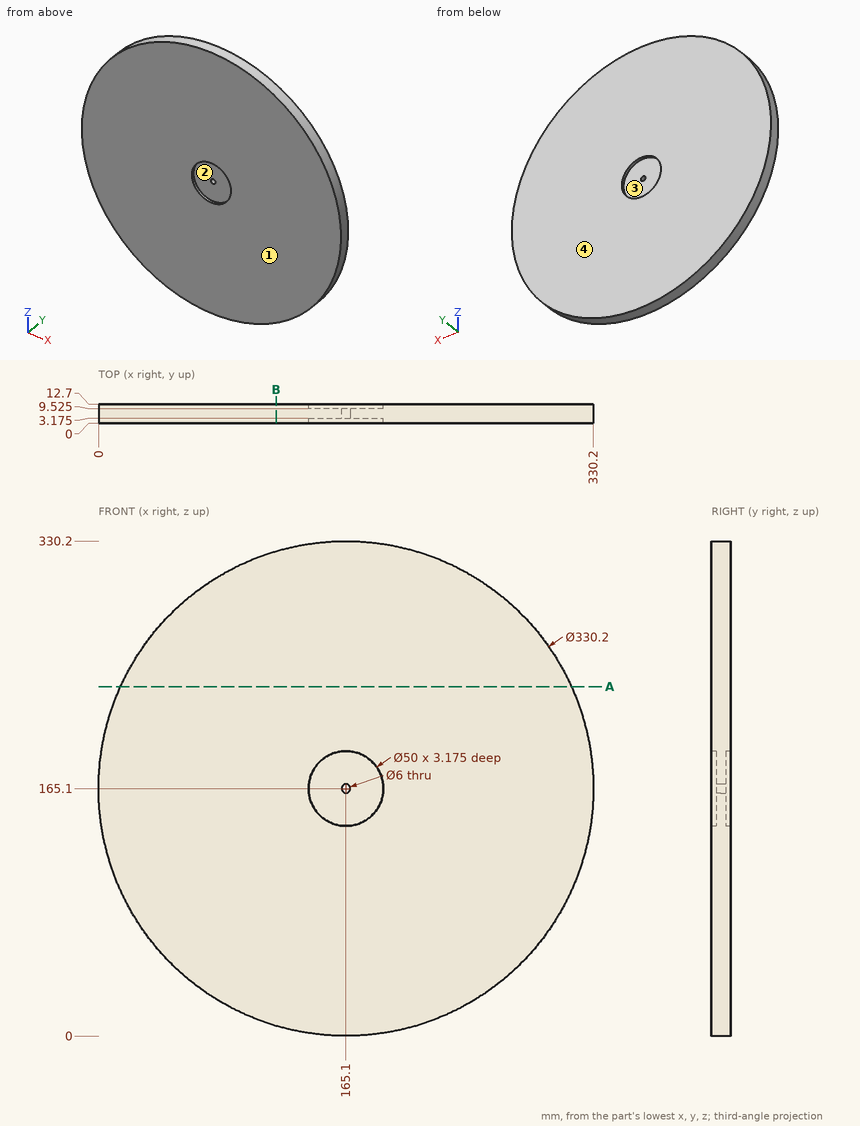
Part print with two shaded views. Sizes in mm from the minimum x, y, z corner. A direction names the side the tool comes from. Round coordinates to 2 decimals unless told otherwise and drop trailing zeros. Write each loop counter-clockwise with the first axis right and the second up, starting at its lowest first coordinate (ties: lowest second). Pieces come first, ordered by that corner, then holes. Notation, with made-up numbers: M -6,45 L 16,45 A25 cw 16,83 Z; hole C -13,-32 d7. An arc over 180 degrees is marked long. Put each result on its own line as item: value. Start each with the question number.
1) Pull direction X, two halves, no side cores. Call the marked faces 3 and 4: pulls with the +X half, pulls with the -X half, needs draft (parallel to the pull), parting line crosses it, or undercut.
2) Drill centre lines: probe 1 along X at (y, z) = (10.5, 165.1); probe 2 along X at (y, z) = (7.75, 165.1); probe 3 along Z at (x, y) = (216, 2). Where is each one in solid material? Low to high. Write a range as [from, to].
3) Pin check, flat tips, straight feed: pin 1 Ø6 at (y, z) = (2, 140.5) entering from +X; pin 2 Ø5 at (x, y) = (194.5, 4) entering from +Z; pin 3 Ø6 at (x, y) = (191.5, 3.5) entering from +Z; pin 4 Ø5.5 at (x, z) = (165.1, 165.1) entering from +Y. Stop position of each tip, or through.
4) Saw through at A-A, the plane z = 233. Write the cut outline in (x, y).
5) 3-axis set-ups, long thin cutter, end or side, ignore diameter. For the marked faces 1 and 2: which of +Z, -Z, +X, -X, +Y, -Y reach the whole face in a straight line?
6) Saw through at B-B, the plane x = 118.5. Write the cut outline in (y, z).
Resolved:
1. face 3: undercut
1. face 4: needs draft
2. probe 1: [0, 140.1], [190.1, 330.2]
2. probe 2: [0, 162.1], [168.1, 330.2]
2. probe 3: [8.04, 322.16]
3. pin 1: x = 328.78
3. pin 2: z = 327.99
3. pin 3: z = 328.53
3. pin 4: through
4. outline: M 14.61,0 L 315.59,0 L 315.59,12.7 L 14.61,12.7 Z
5. face 1: +Z, -Z, +X, -X, -Y
5. face 2: -Y
6. outline: M 0,6.71 L 12.7,6.71 L 12.7,323.49 L 0,323.49 Z
